from build123d import *

# Parameters (mm, degrees)
F0_W     = 76.2
F0_H     = 63.5
F1_DEPTH = 1.524
F3_DEPTH = 76.2
F5_D     = 4.7625


# Not quite as in the source:
# - a pattern or mirror of a feature is missing from the dataset's text; its kind, count and spacing are read off the source's solid


with BuildPart() as f1:
    # F0 (on Right) → F1 (new body)
    with BuildSketch(Plane.YZ):
        Rectangle(F0_W, F0_H)
    extrude(amount=F1_DEPTH)

    # F2 (on face) → F3 (join, through all)
    with BuildSketch(Plane.XZ.offset(38.1)):
        with BuildLine():
            ThreePointArc((1.524, -2.1552614691), (3.6058227154, -1.866511184), (4.572, 0))
            ThreePointArc((4.572, 0), (3.6058227154, 1.866511184), (1.524, 2.1552614691))
            Line((1.524, 2.1552614691), (1.524, -2.1552614691))
        make_face()
    extrude(amount=-F3_DEPTH)

    # F5 (through all)
    with Locations(Plane.YZ.offset(1.524)):
        with Locations((-30.1625, 19.05), (0, 23.8125), (30.1625, 19.05)):
            f5 = Hole(F5_D / 2)

    # F5_copies: F5 across plane
    add(f5.mirror(Plane(origin=(0, 0, 0), x_dir=(-1, 0, 0), z_dir=(0, 0, -1))), mode=Mode.SUBTRACT)


solid = f1.part
Read the model definition and answer for the solid it produces. Units are mm, in the model's axes. Round coordinates to 2 decimals unless told otherwise and drop trailing zeros. Write each loop counter-clockwise with the first axis right and the second up, starting at its lowest first coordinate (ties: lowest second). Pieces come first, ordered by that corner, then holes. Notation, with made-up numbers: (81.5, 19.25) - (114.5, 19.25) arc R35 ccw to (114.5, 53.25) - close; hole circle Ø2 at (81.25, 88). An arc over 180 degrees is marked (long way). One line per question, with ' | ' between items. Start each with the question number.
1. Section A-A (z = 19.05) is taken. Determine the outline of the cut face in (x, y).
2. Find the intervals of material crossed by probe 1 along Z at (x, y) = (1.15, 0); probe 2 along Z at (x, y) = (1.1, 28.5); probe 3 along X at (y, z) = (-3, -8), in increasing order. Write a range as [from, to].
3. This flat-tipped pin is pushed along its axis until it touches: pin 1 (9 mm diameter, centred on y = 16.5, z = 18.5, fed in from +X). Where does it stop, or does it pass through?
4. Section D-D (y = 26.5) is taken. Determine the outline of the cut face in (x, z), and give its area (3 significant figures).
5. Section C-C (x = 0.75) is taken. Determine the outline of the cut face in (y, z), and give its area (3 significant figures).
6. Section B-B (y = 0) is taken. Determine the outline of the cut face in (x, z), and give its area (3 significant figures).
7. For a pull along Z with two mould halves and no side action, classify faces 1 (the face through (1, -1, 31.75)), 2 (the face through (1.524, -1, 17)), 3 (the face through (0.75, 32.54, 19.15)), 4 (the face through (0.75, 32.54, -19.15)) as +Z half, -Z half, draft (parallel to the pull), parting line (faces both ways), or undercut.
Filled in:
1) outline: (0, -38.1) - (1.52, -38.1) - (1.52, -32.54) - (0, -32.54) - close; (0, -27.78) - (1.52, -27.78) - (1.52, 27.78) - (0, 27.78) - close; (0, 32.54) - (1.52, 32.54) - (1.52, 38.1) - (0, 38.1) - close
2) probe 1: [-31.75, -26.19], [-21.43, 21.43], [26.19, 31.75] | probe 2: [-31.75, -20.75], [-17.35, 17.35], [20.75, 31.75] | probe 3: [0, 1.52]
3) pin 1: x = 1.52
4) outline: (0, -31.75) - (1.52, -31.75) - (1.52, -2.16) arc R2.29 ccw (long way) to (1.52, 2.16) - (1.52, 31.75) - (0, 31.75) - close | area: 108 mm²
5) outline: (-38.1, -31.75) - (38.1, -31.75) - (38.1, 31.75) - (-38.1, 31.75) - close; hole circle Ø4.76 at (-30.16, -19.05); hole circle Ø4.76 at (-30.16, 19.05); hole circle Ø4.76 at (0, -23.81); hole circle Ø4.76 at (0, 23.81); hole circle Ø4.76 at (30.16, -19.05); hole circle Ø4.76 at (30.16, 19.05) | area: 4,730 mm²
6) outline: (0, -31.75) - (1.52, -31.75) - (1.52, -26.19) - (0, -26.19) - close; (0, -21.43) - (1.52, -21.43) - (1.52, -2.16) arc R2.29 ccw (long way) to (1.52, 2.16) - (1.52, 21.43) - (0, 21.43) - close; (0, 26.19) - (1.52, 26.19) - (1.52, 31.75) - (0, 31.75) - close | area: 93.9 mm²
7) face 1: +Z half | face 2: draft | face 3: undercut | face 4: undercut
